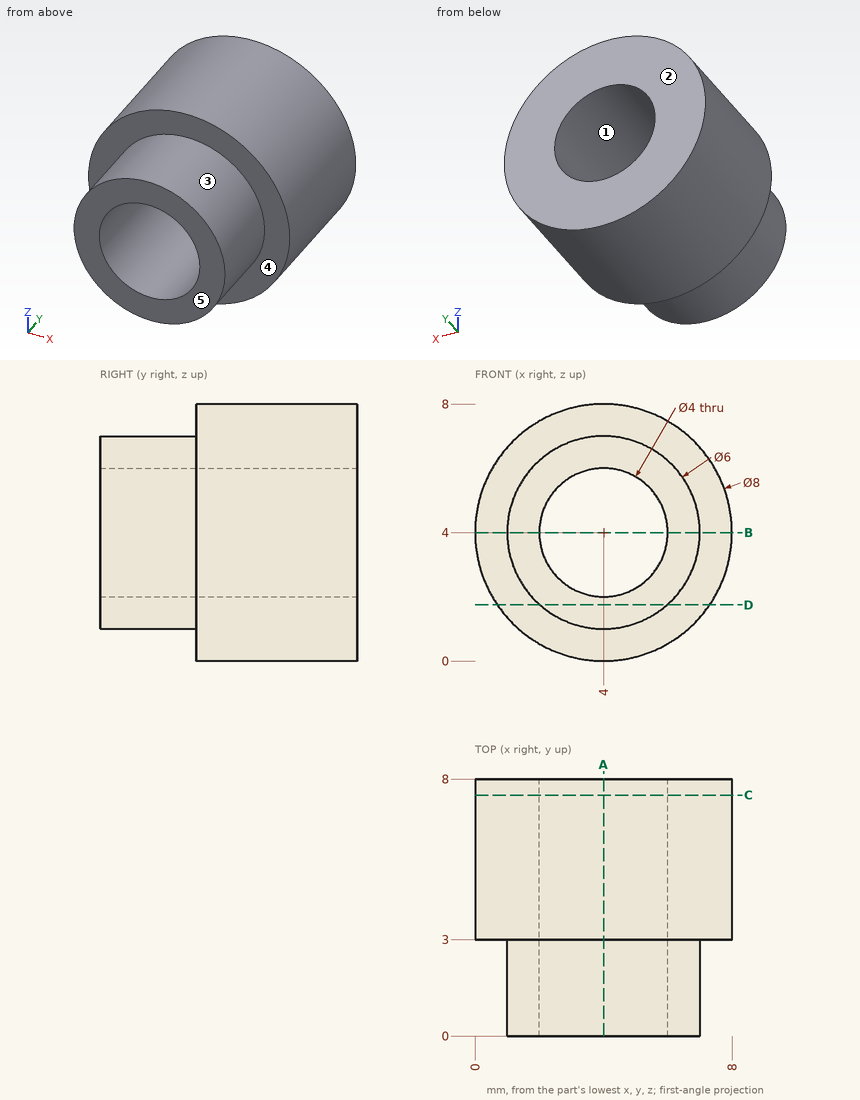
Print and shaded views of the part. All mm, measured from the part's lowest x, y and z. A direction names the side the tool comes from. Give positions to 0.01 mm unless a question says otherwise; leave off trailing zeros. Loops run counter-clockwise (first coordinate to the right, second up) from the corner with the lowest first, then second, coordinate; pieces in that order, holes last.
1) Pull direction Z, two halves, no side cores. Call the marked faces 1, 2 and 3: +Z half, -Z half, draft (parallel to the pull), parting line (faces both ways), or undercut.
2) Flat gauge pins, fed straight in: pin 1 Ø2 at (x, y) = (4, 1.5) entering from +Z; pin 2 Ø1.5 at (x, y) = (1, 2.5) entering from -Z; pin 3 Ø3 at (x, y) = (7, 2.5) entering from +Z; pin 4 Ø4 at (x, z) = (3, 1.5) entering from -Y. Where does each tip first touch, or does it go through?
3) Tool access for the marked faces 4 and 5: list every direction of +Z, -Z, +X, -X, +Y, -Y with a clear straight run to the whole face (end or side of a thin tool).
4) Wall check: line 1 (Z direction, x = 4, y = 3.5); line 2 (Z direction, x = 4, y = 1.5); line 3 (Y direction, x = 0.5, z = 4.75). Give the ranges that are in metal, low to high.
5) Saw through at D-D (z = 1.75). Write the cut outline in (x, y).
6) Saw through at A-A (x = 4). Write the cut outline in (y, z), plus the area to 3 significant figures.
7) Saw through at C-C (y = 7.5). Write the cut outline in (x, z), plus the area to 3 significant figures.
8) Saw through at B-B (z = 4). Write the cut outline in (x, y).
Answer block:
1. face 1: undercut
1. face 2: draft
1. face 3: parting line
2. pin 1: stops at z = 7
2. pin 2: stops at z = 0.83
2. pin 3: stops at z = 7.67
2. pin 4: stops at y = 0
3. face 4: -Y
3. face 5: +Z, -Z, +X, -X, -Y
4. line 1: z = 0 to 2, 6 to 8
4. line 2: z = 1 to 2, 6 to 7
4. line 3: y = 3 to 8
5. outline: (0.69, 3) - (2.02, 3) - (2.02, 0) - (5.98, 0) - (5.98, 3) - (7.31, 3) - (7.31, 8) - (0.69, 8) - close
6. outline: (0, 1) - (3, 1) - (3, 0) - (8, 0) - (8, 2) - (0, 2) - close; (0, 6) - (8, 6) - (8, 8) - (3, 8) - (3, 7) - (0, 7) - close
6. area: 26.0 mm2
7. outline: circle Ø8 at (4, 4); hole circle Ø4 at (4, 4)
7. area: 37.7 mm2
8. outline: (0, 3) - (1, 3) - (1, 0) - (2, 0) - (2, 8) - (0, 8) - close; (6, 0) - (7, 0) - (7, 3) - (8, 3) - (8, 8) - (6, 8) - close
